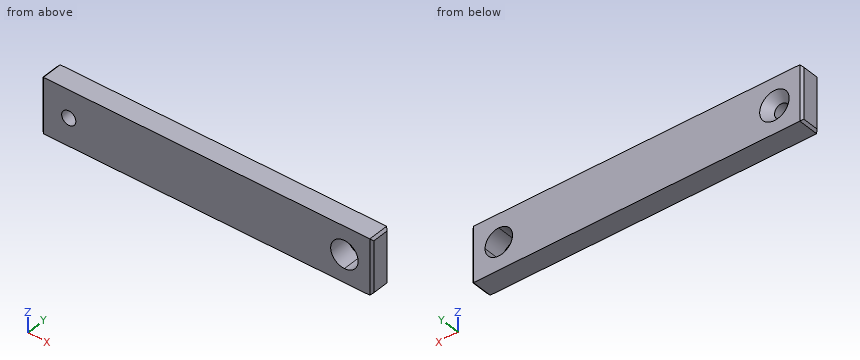
```python
from build123d import *

# Parameters (mm, degrees)
SKETCH1_W                                         = 76.2
SKETCH1_H                                         = 12.7
BOSS_EXTRUDE2_DEPTH                               = 4.7625
CSK_FOR_4_FLAT_HEAD_SOCKET_CAP_SCREW1_D           = 3.2639
CSK_FOR_4_FLAT_HEAD_SOCKET_CAP_SCREW1_CSINK_D     = 6.7818
CSK_FOR_4_FLAT_HEAD_SOCKET_CAP_SCREW1_CSINK_ANGLE = 82
CUT_EXTRUDE1_DEPTH                                = 5.7625
CHAMFER1_SIZE                                     = 0.508


with BuildPart() as part:
    # Sketch1 → Boss-Extrude2 (new body)
    with BuildSketch(Plane(origin=(0, 0, 0), x_dir=(1, 0, 0), z_dir=(0, 1, 0))):
        with Locations((-31.75, 0)):
            Rectangle(SKETCH1_W, SKETCH1_H)
    extrude(amount=BOSS_EXTRUDE2_DEPTH)

    # CSK for #4 Flat Head Socket Cap Screw1 (through all)
    with Locations(Plane(origin=(0, 4.7625, 0), x_dir=(1, 0, 0), z_dir=(0, 1, 0))):
        with Locations((-63.5, 0)):
            CounterSinkHole(CSK_FOR_4_FLAT_HEAD_SOCKET_CAP_SCREW1_D / 2, CSK_FOR_4_FLAT_HEAD_SOCKET_CAP_SCREW1_CSINK_D / 2, counter_sink_angle=CSK_FOR_4_FLAT_HEAD_SOCKET_CAP_SCREW1_CSINK_ANGLE)

    # Sketch2 → Cut-Extrude1 (cut, through all)
    with BuildSketch(Plane(origin=(0, 4.7625, 0), x_dir=(1, 0, 0), z_dir=(0, 1, 0))):
        with BuildLine():
            ThreePointArc((3.1623, 0), (2.236083774, 2.236083774), (0, 3.1623))
            Line((0, 3.1623), (0, -3.1623))
            ThreePointArc((0, -3.1623), (2.236083774, -2.236083774), (3.1623, 0))
        make_face()
        with BuildLine():
            Line((0, -3.1623), (0, 3.1623))
            ThreePointArc((0, 3.1623), (-3.1623, 0), (0, -3.1623))
        make_face()
    extrude(amount=-CUT_EXTRUDE1_DEPTH, mode=Mode.SUBTRACT)

    # Chamfer1
    chamfer1_edges = [part.edges().sort_by_distance(p)[0] for p in [
        (-69.85, 2.38125, 6.35),
        (-69.85, 2.38125, -6.35),
        (6.35, 2.38125, -6.35),
        (6.35, 2.38125, 6.35),
        (6.35, 4.7625, 0),
        (-69.85, 4.7625, 0),
        (-69.85, 0, 0),
        (6.35, 0, 0),
    ]]
    chamfer(chamfer1_edges, length=CHAMFER1_SIZE)


solid = part.part
```
Geometry: final body of the model. Coordinates: model frame, mm. Round coordinates to 2 decimals unless told otherwise and drop trailing zeros. Write each loop counter-clockwise with the first axis right and the second up, starting at its lowest first coordinate (ties: lowest second). Pieces come first, ordered by that corner, then holes.
Item 1: Material intervals for L1, parallel to Z at x = -63.5, y = 2.15; L2, parallel to X at y = 1.7, z = 2.5; L3, parallel to Z at x = -1.5, y = 2, sorted ascending.
Item 2: Pin query (flat end, axial travel): P1, Ø1.5, axis at x = -7.5, z = -5, coming from the -Y side. Return the tip coordinate at first contact, or that it passes through.
Item 3: Section query A-A (x = -63.5). Return loops of the section in (y, z), plus the area to 3 significant figures.
Completed:
1. L1: z = -6.35 to -1.63, 1.63 to 6.35
1. L2: x = -69.85 to -1.94, 1.94 to 6.35
1. L3: z = -6.35 to -2.78, 2.78 to 6.35
2. P1: stops at y = 0
3. outline: (0, -6.35) - (4.76, -6.35) - (4.76, -3.39) - (2.74, -1.63) - (0, -1.63) - close; (0, 1.63) - (2.74, 1.63) - (4.76, 3.39) - (4.76, 6.35) - (0, 6.35) - close
3. area: 41.4 mm2
